Check sheet for the modelled part. Datum: model origin and axes. Units: mm. Round coordinates to 2 decimals unless told otherwise and drop trailing zeros. Write each loop counter-clockwise with the first axis right and the second up, starting at its lowest first coordinate (ties: lowest second). Pieces come first, ordered by that corner, then holes.
Item 1: Section check B-B, the plane x = 69. Record the cut outline in (y, z), plus the area to 3 significant figures.
Item 2: Material ranges on line 1 along X through (y, z) = (6.25, 175); line 2 along X through (y, z) = (12.25, 115); line 3 along Z through (x, y) = (95.5, 10.75), recorded low to high.
Item 3: Section check A-A, the plane y = 8.5. Record the cut outline in (x, z).
Item 4: Release check for a two-part mould opening along X. For faces 1 (the flat face through (-1, 19, 129)), 2 (the conical face through (96.372, 16.621, 206.367)), 3 (the flat face through (53, 9, 272)) record: pulls with the +X half, pulls with the -X half, needs draft (parallel to the pull), parting line crosses it, or undercut.
Item 5: Section check C-C, the plane x = 38.5. Record the cut outline in (y, z), plus the area to 3 significant figures.
Item 6: Depth check by flat-ended pin: pin 1 (10 mm diameter, centred on x = 25.5, y = 11, fed in from +Z); pin 2 (8 mm diameter, centred on x = 31.5, y = 12.5, fed in from +Z); pin 3 (4 mm diameter, centred on x = -25, y = 3, fed in from +Z). Enter the tip coordinate at first touch or a pass-through.
from build123d import *

# Parameters (mm, degrees)
F1_DEPTH       = 19
F3_D           = 3
F3_CSINK_D     = 8
F3_CSINK_ANGLE = 90
F4_D           = 4.4


with BuildPart() as f1:
    # F0 (on Front) → F1 (new body)
    with BuildSketch(Plane.XZ):
        Polygon((-105, 0), (105, 0), (105, 220), (0, 325), (-105, 220), align=None)
    extrude(amount=-F1_DEPTH)

    # F3 (through all)
    with Locations(Plane(origin=(0, 19, 0), x_dir=(-1, 0, 0), z_dir=(0, 1, 0))):
        with Locations((-95.5, 25), (-95.5, 115), (-95.5, 205), (76.5, 175)):
            CounterSinkHole(F3_D / 2, F3_CSINK_D / 2, counter_sink_angle=F3_CSINK_ANGLE)

    # F4 (through all)
    with Locations(Plane(origin=(0, 19, 0), x_dir=(-1, 0, 0), z_dir=(0, 1, 0))):
        with Locations((95.5, 210.5)):
            Hole(F4_D / 2)


solid = f1.part
Values found:
1. outline: (0, 0) - (19, 0) - (19, 256) - (0, 256) - close
1. area: 4,860 mm2
2. line 1: x = -105 to -78, -75 to 105
2. line 2: x = -105 to 94, 97 to 105
2. line 3: z = 0 to 23.5, 26.5 to 113.5, 116.5 to 203.5, 206.5 to 229.5
3. outline: (-105, 0) - (105, 0) - (105, 220) - (0, 325) - (-105, 220) - close; hole circle Ø4.4 at (-95.5, 210.5); hole circle Ø3 at (-76.5, 175); hole circle Ø3 at (95.5, 25); hole circle Ø3 at (95.5, 115); hole circle Ø3 at (95.5, 205)
4. face 1: needs draft
4. face 2: undercut
4. face 3: pulls with the +X half
5. outline: (0, 0) - (19, 0) - (19, 286.5) - (0, 286.5) - close
5. area: 5,440 mm2
6. pin 1: stops at z = 304.5
6. pin 2: stops at z = 297.5
6. pin 3: stops at z = 302
